from build123d import *

# Parameters (mm, degrees)
SKETCH1_W                   = 50
SKETCH1_H                   = 50
BOSS_EXTRUDE1_DEPTH         = 3.2
F_1_4_CLEARANCE_SLOT2_DEPTH = 3.2


# Read off the part's stored shape, not the designer's step: 1/4 Clearance Slot2
with BuildPart() as part:
    # Sketch1 → Boss-Extrude1 (new body)
    with BuildSketch(Plane(origin=(0, 0, 0), x_dir=(1, 0, 0), z_dir=(0, 1, 0))):
        Rectangle(SKETCH1_W, SKETCH1_H)
    extrude(amount=BOSS_EXTRUDE1_DEPTH)

    # 1/4 Clearance Slot2 outline → 1/4 Clearance Slot2 (cut)
    with BuildSketch(Plane(origin=(0, 0, 0), x_dir=(1, 0, 0), z_dir=(0, 1, 0))):
        with BuildLine():
            Line((-3.175, -3.2639), (3.175, -3.2639))
            ThreePointArc((3.175, -3.2639), (6.4389, 0), (3.175, 3.2639))
            Line((3.175, 3.2639), (-3.175, 3.2639))
            ThreePointArc((-3.175, 3.2639), (-6.4389, 0), (-3.175, -3.2639))
        make_face()
    extrude(amount=F_1_4_CLEARANCE_SLOT2_DEPTH, mode=Mode.SUBTRACT)


solid = part.part
Model file for the job. Use its own axes, mm. A direction names the side the tool comes from. Give positions to 0.01 mm unless a question says otherwise; leave off trailing zeros. Loops run counter-clockwise (first coordinate to the right, second up) from the corner with the lowest first, then second, coordinate; pieces in that order, holes last.
Item 1: Drill centre lines: line 1 along Z through (x, y) = (1.5, 0.7); line 2 along X through (y, z) = (0.65, -1); line 3 along X through (y, z) = (1.75, -1.5). Where is each one in solid material? Low to high.
Check values:
line 1: z = -25 to -3.26, 3.26 to 25
line 2: x = -25 to -6.28, 6.28 to 25
line 3: x = -25 to -6.07, 6.07 to 25
Item 2: Which spindle directions (+Z, -Z, +X, -X, +Y, -Y) get a long thin tool onto all of the face, cutting with end or side? Do faces 4 (the face through (-25, 2, 0)), 5 (the face through (0, 2, 3.264)). Say none if no direction does.
Check values:
face 4: +Z, -Z, -X, +Y, -Y
face 5: +Y, -Y
Item 3: Slice it at A-A (z = 0). Write the cut outline in (x, y).
Check values:
outline: (-25, 0) - (-6.44, 0) - (-6.44, 3.2) - (-25, 3.2) - close; (6.44, 0) - (25, 0) - (25, 3.2) - (6.44, 3.2) - close
Item 4: Slice it at C-C (y = 0.55). Write the cut outline in (x, z) (3 decimals).
Check values:
outline: (-25, -25) - (25, -25) - (25, 25) - (-25, 25) - close; hole (-3.175, -3.264) - (3.175, -3.264) arc R3.264 ccw to (3.175, 3.264) - (-3.175, 3.264) arc R3.264 ccw to start
Item 5: Mould opens along Z. For faces 1 (the face through (0, 2, -25)), 2 (the face through (25, 2, 0)), 3 (the face through (-6.44, 1.58, -0.07)) say: +Z half, -Z half, draft (parallel to the pull), parting line (faces both ways), or undercut.
Check values:
face 1: -Z half
face 2: draft
face 3: undercut
Item 6: Slice it at B-B (x = 0.5). Write the cut outline in (y, z).
Check values:
outline: (0, -25) - (3.2, -25) - (3.2, -3.26) - (0, -3.26) - close; (0, 3.26) - (3.2, 3.26) - (3.2, 25) - (0, 25) - close
